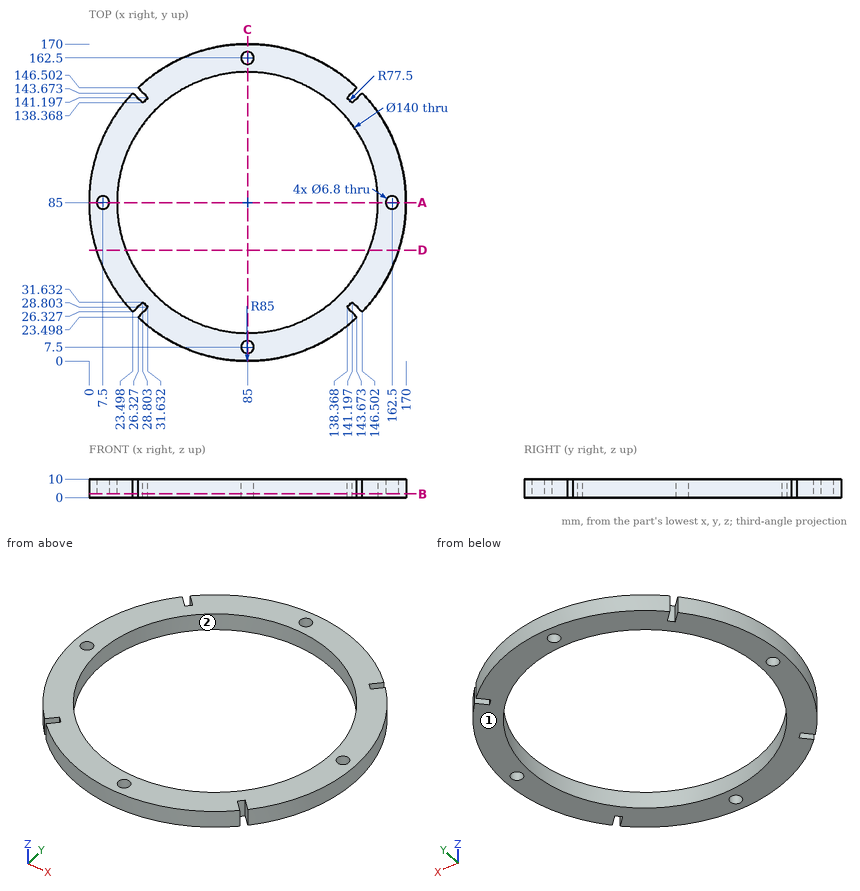
Could you check a few things on this drawing? It's one solid part, dimensions in mm from its lowest x, y, z. Give positions to 0.01 mm unless a question says otherwise; leave off trailing zeros. Order: outer loops, then holes, each group sorted by start corner. A loop starts at its lowest first (then second) coordinate and runs counter-clockwise, first axis right, second up. Notation, with made-up numbers: (19.25, -35) - (47.25, -35) arc R24 ccw to (47.25, -4) - close; hole circle Ø7 at (24.25, -36.75). An arc over 180 degrees is marked (long way). Answer as a JSON object with one key per item and string values. Group by question number.
Item 1: Please list where these lines run through material, in increasing order: probe 1 along Y at (x, z) = (85, 5); probe 2 along Y at (x, z) = (112, 6.5); probe 3 along Y at (x, z) = (7.5, 3).
Item 2: If we section it at A-A on y = 85: Please give me the cut outline in (x, z).
Item 3: For P1, Ø1, axis at y = 21.5, z = 7, coming from the -X side; P2, Ø4, axis at y = 127, z = 2, coming from the -X side; P3, Ø5, axis at x = 139, z = 5, coming from the +Y side, each with a flat end and sliding along its axis, tell me the tip position at first contact or that it passes through.
Item 4: If we section it at D-D on y = 59.5: Please give me the cut outline in (x, z) (1 decimal).
Item 5: If we section it at B-B on z = 2: Please give me the cut outline in (x, y).
Item 6: If we mould it in two halves opening along X, with no side actions, what happens to the marked faces 1 and 2? For each: pulls with the +X half, pulls with the -X half, needs draft (parallel to the pull), parting line crosses it, or undercut.
Result set:
{
 "1": {"probe 1": "0 to 4.1, 10.9 to 15, 155 to 159.1, 165.9 to 170", "probe 2": "4.4 to 20.42, 149.58 to 165.6", "probe 3": "50.09 to 81.6, 88.4 to 119.91"},
 "2": {"outline": "(0, 0) - (4.1, 0) - (4.1, 10) - (0, 10) - close; (10.9, 0) - (15, 0) - (15, 10) - (10.9, 10) - close; (155, 0) - (159.1, 0) - (159.1, 10) - (155, 10) - close; (165.9, 0) - (170, 0) - (170, 10) - (165.9, 10) - close"},
 "3": {"P1": "x = 27.94", "P2": "x = 10", "P3": "y = 152.62"},
 "4": {"outline": "(3.9, 0) - (19.8, 0) - (19.8, 10) - (3.9, 10) - close; (150.2, 0) - (166.1, 0) - (166.1, 10) - (150.2, 10) - close"},
 "5": {"outline": "(23.5, 26.33) - (28.8, 31.63) arc R77.5 ccw to (31.63, 28.8) - (26.33, 23.5) arc R85 ccw to (143.67, 23.5) - (138.37, 28.8) arc R77.5 ccw to (141.2, 31.63) - (146.5, 26.33) arc R85 ccw to (146.5, 143.67) - (141.2, 138.37) arc R77.5 ccw to (138.37, 141.2) - (143.67, 146.5) arc R85 ccw to (26.33, 146.5) - (31.63, 141.2) arc R77.5 ccw to (28.8, 138.37) - (23.5, 143.67) arc R85 ccw to start; hole circle Ø6.8 at (7.5, 85); hole circle Ø140 at (85, 85); hole circle Ø6.8 at (85, 7.5); hole circle Ø6.8 at (85, 162.5); hole circle Ø6.8 at (162.5, 85)"},
 "6": {"face 1": "needs draft", "face 2": "undercut"}
}
